CAD build for the part. Positions are in the model's coordinates, mm. A direction names the side the tool comes from. Coordinates: 2 decimals unless noted, no trailing zeros. Loops run counter-clockwise (first coordinate to the right, second up) from the corner with the lowest first, then second, coordinate; pieces in that order, holes last. Notation, with made-up numbers: M -33.75,6 L -3.75,6 A13 ccw -3.75,15 Z; hole C -23,-28 d3. An arc over 180 degrees is marked long. Answer as a JSON object with one key per item and string values. Group by question number.
```python
from build123d import *

# Parameters (mm, degrees)
SKETCH1_W                      = 32
SKETCH1_H                      = 32
BOSS_EXTRUDE1_DEPTH            = 32
SKETCH2_W                      = 28
SKETCH2_H                      = 30
CUT_EXTRUDE1_DEPTH             = 33
F_8_0_8_DIAMETER_HOLE1_D       = 8
F_8_0_8_DIAMETER_HOLE1_DEPTH   = 2
F_3_7_3_7_DIAMETER_HOLE1_D     = 3.7
F_3_7_3_7_DIAMETER_HOLE1_DEPTH = 2
F_3_7_3_7_DIAMETER_HOLE2_D     = 3.7
F_3_7_3_7_DIAMETER_HOLE2_DEPTH = 2
F_8_0_8_DIAMETER_HOLE2_D       = 8
F_8_0_8_DIAMETER_HOLE2_DEPTH   = 32
F_8_0_8_DIAMETER_HOLE3_D       = 8
F_8_0_8_DIAMETER_HOLE3_DEPTH   = 32
F_3_7_3_7_DIAMETER_HOLE3_D     = 3.7
F_3_7_3_7_DIAMETER_HOLE3_DEPTH = 32
FILLET1_R                      = 2.5


with BuildPart() as part:
    # Sketch1 → Boss-Extrude1 (new body)
    with BuildSketch(Plane(origin=(16, 0, 0), x_dir=(0, 0, -1), z_dir=(1, 0, 0))):
        with Locations((0, 16)):
            Rectangle(SKETCH1_W, SKETCH1_H)
    extrude(amount=-BOSS_EXTRUDE1_DEPTH)

    # Sketch2 → Cut-Extrude1 (cut, through all)
    with BuildSketch(Plane(origin=(0, 0, -16), x_dir=(-1, 0, 0), z_dir=(0, 0, -1))):
        with Locations((0, 17)):
            Rectangle(SKETCH2_W, SKETCH2_H)
    extrude(amount=-CUT_EXTRUDE1_DEPTH, mode=Mode.SUBTRACT)

    # Ø8.0 (8) Diameter Hole1
    with Locations(Plane.ZY.offset(16)):
        with Locations((0, 16)):
            Hole(F_8_0_8_DIAMETER_HOLE1_D / 2, depth=F_8_0_8_DIAMETER_HOLE1_DEPTH)

    # Ø3.7 (3.7) Diameter Hole1
    with Locations(Plane.ZY.offset(16)):
        with Locations((-8, 16), (0, 24), (8, 16), (0, 8), (-5.656854249, 21.656854249), (5.656854249, 21.656854249), (5.656854249, 10.343145751), (-5.656854249, 10.343145751)):
            Hole(F_3_7_3_7_DIAMETER_HOLE1_D / 2, depth=F_3_7_3_7_DIAMETER_HOLE1_DEPTH)

    # Ø3.7 (3.7) Diameter Hole2
    with Locations(Plane(origin=(0, 2, 0), x_dir=(1, 0, 0), z_dir=(0, 1, 0))):
        with Locations((8, 0), (0, 8), (-8, 0), (0, -8), (5.656854249, 5.656854249), (-5.656854249, 5.656854249), (-5.656854249, -5.656854249), (5.656854249, -5.656854249)):
            Hole(F_3_7_3_7_DIAMETER_HOLE2_D / 2, depth=F_3_7_3_7_DIAMETER_HOLE2_DEPTH)

    # Ø8.0 (8) Diameter Hole2
    with Locations(Plane(origin=(0, 0, 0), x_dir=(-1, 0, 0), z_dir=(0, -1, 0))):
        with Locations((0, 0)):
            Hole(F_8_0_8_DIAMETER_HOLE2_D / 2, depth=F_8_0_8_DIAMETER_HOLE2_DEPTH)

    # Ø8.0 (8) Diameter Hole3
    with Locations(Plane(origin=(16, 0, 0), x_dir=(0, 0, -1), z_dir=(1, 0, 0))):
        with Locations((0, 16)):
            Hole(F_8_0_8_DIAMETER_HOLE3_D / 2, depth=F_8_0_8_DIAMETER_HOLE3_DEPTH)

    # Ø3.7 (3.7) Diameter Hole3
    with Locations(Plane(origin=(16, 0, 0), x_dir=(0, 0, -1), z_dir=(1, 0, 0))):
        with Locations((8, 16), (0, 24), (-8, 16), (0, 8), (5.656854249, 21.656854249), (-5.656854249, 21.656854249), (-5.656854249, 10.343145751), (5.656854249, 10.343145751)):
            Hole(F_3_7_3_7_DIAMETER_HOLE3_D / 2, depth=F_3_7_3_7_DIAMETER_HOLE3_DEPTH)

    # Fillet1
    fillet1_edges = [part.edges().sort_by_distance(p)[0] for p in [
        (-16, 0, 0),
        (15, 32, 16),
        (15, 32, -16),
        (16, 0, 0),
        (-15, 32, -16),
        (-15, 32, 16),
    ]]
    fillet(fillet1_edges, radius=FILLET1_R)


solid = part.part
```
Item 1: Pull direction X, two halves, no side cores. Call faces 3 (the cylindrical face through (-15.248, 0.713, -0.224)), 4 (the cylindrical face through (-14.986, 6.194, 0.401)), 5 (the cylindrical face through (0.401, 0.986, -6.194)), 6 (the cylindrical face through (7.02, 0.986, 4.407)): released by +X, released by -X, zero draft, split by the parting line, or undercut.
Item 2: Drill centre lines: L1, parallel to Z at x = 0, y = 0.45; L2, parallel to X at y = 12.5, z = 3; L3, parallel to Y at x = -0.5, z = -12.5. Where is each one in solid material? Low to high. Write a range as from..to.
Item 3: Pin check, flat tips, straight feed: pin 1 (2 mm diameter, centred on y = 21.66, z = -5.66, fed in from +X); pin 2 (1 mm diameter, centred on x = -8, z = 1.5, fed in from +Y). Stop position of each tip, or through.
Item 4: Tool access for faces 1 (the cylindrical face through (14.986, 6.194, -0.401)), 2 (the flat face through (-14, 20, -4)): list every direction of +Z, -Z, +X, -X, +Y, -Y with a clear straight run to the whole face (end or side of a thin tool).
Item 5: Slice it at D-D, the plane y = 24. Write the cut outline in (x, z).
Item 6: Slice it at A-A, the plane x = -8. Write the cut outline in (y, z), then the cut area to 3 significant figures.
Item 7: Slice it at B-B, the plane y = 16. Count the separate pieces of the cut face and the enclosed holes in it, then the cut area to 3 significant figures.
Item 8: Slice it at C-C, the plane z = -8. Write the cut outline in (x, y), then the cut area to 3 significant figures.
Computed:
{
 "1": {"face 3": "released by -X", "face 4": "zero draft", "face 5": "undercut", "face 6": "undercut"},
 "2": {"L1": "-16..-9.85, -6.15..-4, 4..6.15, 9.85..16", "L2": "-16..-14, 14..16", "L3": "0..2"},
 "3": {"pin 1": "through", "pin 2": "y = 2"},
 "4": {"face 1": "+X, -X", "face 2": "+Z, -Z, +Y"},
 "5": {"outline": "M -16,-16 L -14,-16 L -14,-1.85 L -16,-1.85 Z; M -16,1.85 L -14,1.85 L -14,16 L -16,16 Z; M 14,-16 L 16,-16 L 16,-1.85 L 14,-1.85 Z; M 14,1.85 L 16,1.85 L 16,16 L 14,16 Z"},
 "6": {"outline": "M 0,-16 L 2,-16 L 2,-1.85 L 0,-1.85 Z; M 0,1.85 L 2,1.85 L 2,16 L 0,16 Z", "area": "56.6 mm2"},
 "7": {"separate pieces": "8", "enclosed holes": "0", "area": "66.4 mm2"},
 "8": {"outline": "M -16,2.5 A2.5 ccw -13.5,0 L -1.85,0 L -1.85,2 L -14,2 L -14,14.15 L -16,14.15 Z; M -16,17.85 L -14,17.85 L -14,32 L -16,32 Z; M 1.85,0 L 13.5,0 A2.5 ccw 16,2.5 L 16,14.15 L 14,14.15 L 14,2 L 1.85,2 Z; M 14,17.85 L 16,17.85 L 16,32 L 14,32 Z", "area": "159 mm2"}
}
